Here's how the part is built. I have some questions about the finished solid (model axes, mm). A direction names the side the tool comes from. Coordinates: 2 decimals unless noted, no trailing zeros. Write each loop counter-clockwise with the first axis right and the second up, starting at its lowest first coordinate (ties: lowest second). Pieces come first, ordered by that corner, then holes. Notation, with made-up numbers: M 36.5,48 L 77.5,48 A10 ccw 77.5,52 Z; hole C -20.75,62 d9. An arc over 180 degrees is marked long. Use one line per item in the form item = value. Start each with the question number.
1. I want a section at C-C, the plane x = 164. List the corners of the cut face in (y, z) for me, plus the area to 3 significant figures.
2. I'm going to push flat-ended pins straight in: pin 1 Ø2 at (y, z) = (-10, 72) entering from -X; pin 2 Ø5 at (y, z) = (-16, 55) entering from -X; pin 3 Ø10 at (y, z) = (-4, 129.5) entering from -X. Where does each tip first touch, or does it pass through?
3. I want a section at B-B, the plane y = -20.25. List the corners of the cut face in (x, z) for me, plus the area to 3 significant figures.
4. I want a section at A-A, the plane x = 88.5. List the corners of the cut face in (y, z) for me, plus the area to 3 significant figures.
5. On a 3-axis mill with a long thin cutter (end or side, diameter ignored), from which of +Z, -Z, +X, -X, +Y, -Y can I reach the whole of each face in a straight line? I mean faces 1 (the face through (-178.125, -12.522, 3.758)), 2 (the face through (97, -13, -127)). Say none if no direction works.
6. Please list where these lines run through material, in increasing order: line 1 along Z through (x, y) = (114.5, -13); line 2 along Z through (x, y) = (162, -5.5); line 3 along X through (y, z) = (-9.5, 218). Write a range as [from, to].
7. Thinking about a two-plate mould opening in Z: for faces 3 (the face through (127, -13, -209)), 4 (the face through (70, -13, 177.8)), 5 (the face through (-126.97, -12.52, -2.79)), which applies, released by +Z, released by -Z, zero draft, split by the parting line, or undercut?
8. I want a section at D-D, the plane z = 186.5. List the corners of the cut face in (x, y) for me.
from build123d import *

# Parameters (mm, degrees)
F1_DEPTH = 25.4


with BuildPart() as f1:
    # F0 (on Front) → F1 (new body)
    with BuildSketch(Plane.XZ):
        with BuildLine():
            Line((-11.387531, 177.8), (11.387531, 177.8))
            ThreePointArc((11.387531, 177.8), (0, 178.164295), (-11.387531, 177.8))
        make_face()
        with BuildLine():
            Line((11.387531, -177.8), (-11.387531, -177.8))
            ThreePointArc((-11.387531, -177.8), (0, -178.164295), (11.387531, -177.8))
        make_face()
        with BuildLine():
            Line((127, 241.3), (127, 177.8))
            Line((127, 177.8), (11.387531, 177.8))
            Line((11.387531, 177.8), (-11.387531, 177.8))
            ThreePointArc((-11.387531, 177.8), (-178.164295, 0), (-11.387531, -177.8))
            Line((-11.387531, -177.8), (11.387531, -177.8))
            Line((11.387531, -177.8), (127, -177.8))
            Line((127, -177.8), (127, -241.3))
            Line((127, -241.3), (190.5, -241.3))
            Line((190.5, -241.3), (190.5, -177.8))
            Line((190.5, -177.8), (190.5, -127))
            Line((190.5, -127), (127, -127))
            Line((127, -127), (0, -127))
            ThreePointArc((0, -127), (-127, 0), (0, 127))
            Line((0, 127), (127, 127))
            Line((127, 127), (190.5, 127))
            Line((190.5, 127), (190.5, 177.8))
            Line((190.5, 177.8), (190.5, 241.3))
            Line((190.5, 241.3), (127, 241.3))
        make_face()
    extrude(amount=F1_DEPTH)


solid = f1.part
Answer list:
q1.outline = M -25.4,-241.3 L 0,-241.3 L 0,-127 L -25.4,-127 Z; M -25.4,127 L 0,127 L 0,241.3 L -25.4,241.3 Z
q1.area = 5,810 mm²
q2.pin_1 = -163.41
q2.pin_2 = -170.25
q2.pin_3 = -127.45
q3.outline = M -11.39,-177.8 A178.16 ccw 11.39,-177.8 L 127,-177.8 L 127,-241.3 L 190.5,-241.3 L 190.5,-127 L 0,-127 A127 cw 0,127 L 190.5,127 L 190.5,241.3 L 127,241.3 L 127,177.8 L 11.39,177.8 A178.16 ccw -11.39,177.8 A178.16 ccw Z
q3.area = 52,000 mm²
q4.outline = M -25.4,-177.8 L 0,-177.8 L 0,-127 L -25.4,-127 Z; M -25.4,127 L 0,127 L 0,177.8 L -25.4,177.8 Z
q4.area = 2,580 mm²
q5.face_1 = -X, +Y, -Y
q5.face_2 = +X, +Y, -Y
q6.line_1 = [-177.8, -127], [127, 177.8]
q6.line_2 = [-241.3, -127], [127, 241.3]
q6.line_3 = [127, 190.5]
q7.face_3 = zero draft
q7.face_4 = released by +Z
q7.face_5 = undercut
q8.outline = M 127,-25.4 L 190.5,-25.4 L 190.5,0 L 127,0 Z
